from build123d import *

# Parameters (mm, degrees)
F0_W     = 3
F0_H     = 20
F0_W_2   = 20
F0_H_2   = 3
F1_DEPTH = 3


with BuildPart() as f1:
    # F0 (on Right) → F1 (new body)
    with BuildSketch(Plane.YZ):
        Polygon((17, 10), (17, 21), (-17, 21), (-17, 10), (-17, -10), (-17, -21), (-10, -21), (10, -21), (17, -21), (17, -10), align=None)
        with Locations((18.5, 0)):
            Rectangle(F0_W, F0_H)
        with Locations((-18.5, 0)):
            Rectangle(F0_W, F0_H)
        with Locations((0, -22.5)):
            Rectangle(F0_W_2, F0_H_2)
    extrude(amount=F1_DEPTH)


solid = f1.part
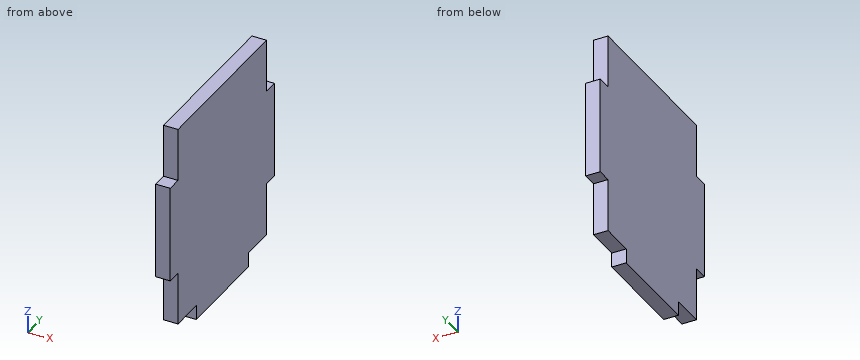
Read the model definition and answer for the solid it produces. Units are mm, in the model's axes. Round coordinates to 2 decimals unless told otherwise and drop trailing zeros. Write each loop counter-clockwise with the first axis right and the second up, starting at its lowest first coordinate (ties: lowest second). Pieces come first, ordered by that corner, then holes.
1. The part is cut by section C-C, the plane y = 15.5. Determine the outline of the cut face in (x, z), then the cut area to 3 significant figures.
2. Given pin 1 Ø0.9 at (x, z) = (1, -22) entering from +Y; pin 2 Ø1.5 at (x, y) = (2, 18) entering from +Z; pin 3 Ø0.9 at (x, y) = (1.5, 19) entering from -Z; pin 4 Ø1 at (y, z) = (12, 0) entering from -X, each flat-ended and moving along its own axis, determine where each tip first touches the part or whether it passes through.
3. The part is cut by section B-B, the plane z = -20. Determine the outline of the cut face in (x, y).
4. Straight lines are drawn through the part: L1, parallel to Y at x = 0.2, z = -12.5; L2, parallel to Z at x = 1.65, y = -15; L3, parallel to Z at x = 2.7, y = 18. For each, find the intervals that lie inside material, in ascending order.
5. The part is cut by section A-A, the plane x = 1.1. Determine the outline of the cut face in (y, z).
Values:
1. outline: (0, -21) - (3, -21) - (3, 21) - (0, 21) - close
1. area: 126 mm2
2. pin 1: stops at y = 10
2. pin 2: stops at z = 10
2. pin 3: stops at z = -10
2. pin 4: stops at x = 0
3. outline: (0, -17) - (3, -17) - (3, 17) - (0, 17) - close
4. L1: y = -17 to 17
4. L2: z = -21 to 21
4. L3: z = -10 to 10
5. outline: (-20, -10) - (-17, -10) - (-17, -21) - (-10, -21) - (-10, -24) - (10, -24) - (10, -21) - (17, -21) - (17, -10) - (20, -10) - (20, 10) - (17, 10) - (17, 21) - (-17, 21) - (-17, 10) - (-20, 10) - close
